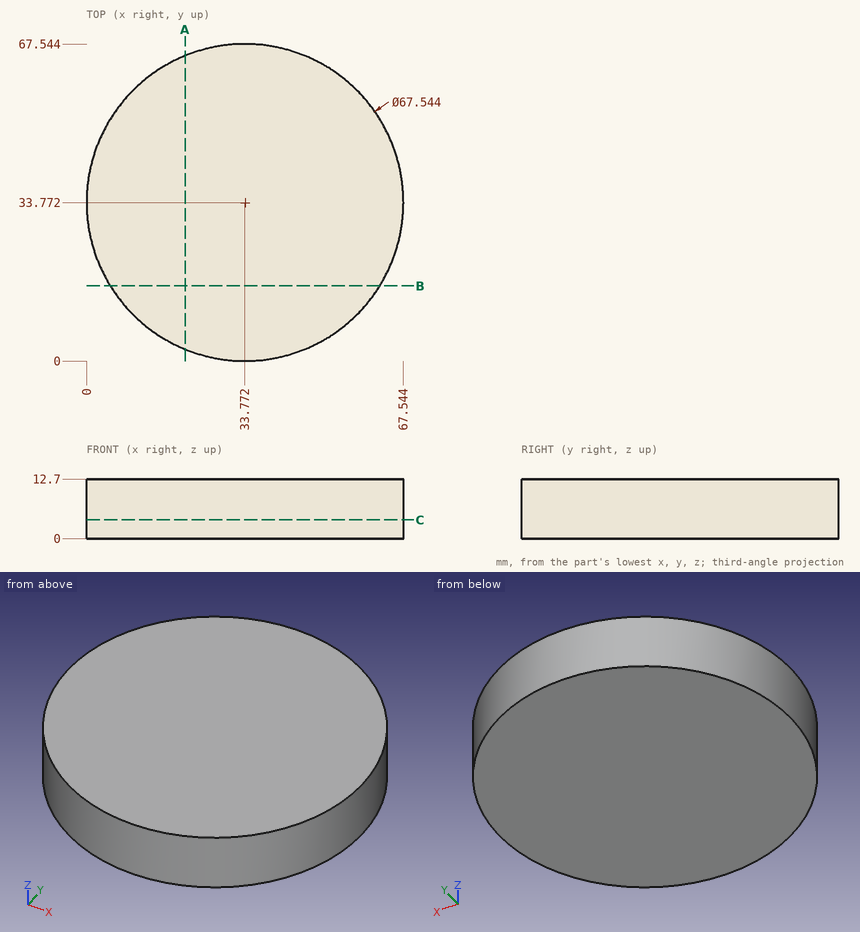
Here's the drawing with two shaded views (mm, measured from the low corner). I have some questions. Give positions to 0.01 mm unless a question says otherwise; leave off trailing zeros. Order: outer loops, then holes, each group sorted by start corner. A loop starts at its lowest first (then second) coordinate and runs counter-clockwise, first axis right, second up. Notation, with made-up numbers: (62.5, 62.5) - (87.5, 62.5) arc R15 ccw to (87.5, 66.5) - close; hole circle Ø1 at (83.5, -11). An arc over 180 degrees is marked (long way). Use a Markdown table: item, result. Add a question column.
Q1. Please list where these lines run through material, in increasing order: line 1 along X through (y, z) = (64.5, 10.5) (1 decimal); line 2 along X through (y, z) = (50.5, 4.75) (1 decimal); line 3 along Y through (x, z) = (10.5, 4) (1 decimal).
Q2. I'm going to push flat-ended pins straight in: pin 1 (1 mm diameter, centred on y = 14, z = 4, fed in from -X); pin 2 (3 mm diameter, centred on x = 39.5, z = 2.5, fed in from -Y); pin 3 (3 mm diameter, centred on y = 21.5, z = 1.5, fed in from -X). Where does each tip first touch, or does it pass through?
Q3. If we section it at A-A on x = 21: Write out the boundary of the cut face in (y, z).
Q4. If we section it at C-C on z = 4: Write out the boundary of the cut face in (x, y), plus the area to 3 significant figures.
Q5. If we section it at B-B on y = 16: Write out the boundary of the cut face in (x, z) (1 decimal).
Answers follow:
| question | item | result |
|---|---|---|
| 1 | line 1 | x = 19.8 to 47.8 |
| 1 | line 2 | x = 4.4 to 63.1 |
| 1 | line 3 | y = 9.3 to 58.2 |
| 2 | pin 1 | stops at x = 6.04 |
| 2 | pin 2 | stops at y = 0.27 |
| 2 | pin 3 | stops at x = 1.76 |
| 3 | outline | (2.51, 0) - (65.04, 0) - (65.04, 12.7) - (2.51, 12.7) - close |
| 4 | outline | circle Ø67.54 at (33.77, 33.77) |
| 4 | area | 3,580 mm^2 |
| 5 | outline | (5.1, 0) - (62.5, 0) - (62.5, 12.7) - (5.1, 12.7) - close |
